Can you work these out from the model? Positions are in its coordinate system, mm. Face numbers are marked on the shaded views. A direction names the side the tool comes from. Round coordinates to 2 decimals unless told otherwise and drop trailing zeros. Loops run counter-clockwise (first coordinate to the right, second up) from the corner with the lowest first, then second, coordinate; pieces in that order, holes last. Notation, with made-up numbers: (-19, -32.5) - (33, -32.5) arc R25 ccw to (33, -9.5) - close; hole circle Ø4 at (-33, 12). An arc over 180 degrees is marked (long way). Answer as CSV lines item,"result".
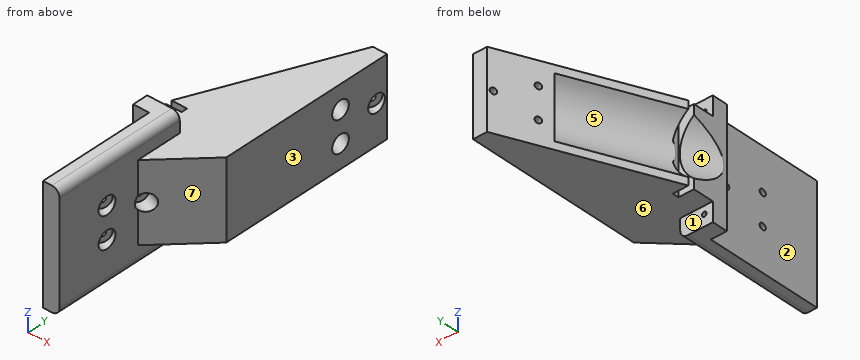
Autodesk Inventor part; units mm, degrees
ref_plane "Work Plane3" through (10.9593, -73.9067, -37.25) normal (-0.9081432, 0.4186597, 0) x (0, 0, 1)
ref_plane "Work Plane4" through (64.6996, 102.2233, -25) normal (-0.9187912, 0.3947439, 0) x (0, 0, 1)
ref_plane "Work Plane5" through (32.5419, 116.0393, -25) normal (-0.9187912, 0.3947439, 0) x (0, 0, 1)
sketch "Sketch1" plane through (0, 0, 0) normal (0, 1, 0) x (-1, 0, 0)
  line L0 (5.5, 37.25) -> (-5.5, 37.25)
  line L1 (-5.5, 37.25) -> (-5.5, -37.25)
  line L2 (-5.5, -37.25) -> (5.5, -37.25)
  line L3 (5.5, -37.25) -> (5.5, 37.25)
  line L4 (5.5, 37.25) -> (-5.5, -37.25) construction
  line L5 (-5.5, 37.25) -> (5.5, -37.25) construction
  circle A0 centre (0, 30) radius 1.5
  line L6 (5.5, 0) -> (-5.5, 0)
  circle A1 centre (0, -30) radius 1.5
  line L7 (-5.5, -25) -> (5.5, -25)
  line L8 (5.5, -25) -> (5.5, 25)
  line L9 (5.5, 25) -> (-5.5, 25)
  line L10 (-5.5, 25) -> (-5.5, -25)
  line L11 (-5.5, -25) -> (5.5, 25) construction
  line L12 (5.5, -25) -> (-5.5, 25) construction
  point P0 (0, 0)
  dimension "d0" = 11
  dimension "d1" = 74.5
  dimension "d2" = 3
  dimension "d3" = 7.25
  dimension "d28" = 50
extrude "Extrusion1" add sketch "Sketch1" along normal blind 10
sketch "Sketch2" plane through (5.5, 0, 37.25) normal (1, 0, 0) x (0, 0, -1)
  line L0 (0, 10) -> (74.5, 10)
  line L1 (0, 0) -> (74.5, 0)
  line L2 (0, 10) -> (74.5, 10)
  line L3 (74.5, 10) -> (74.5, 0)
  line L4 (74.5, 0) -> (0, 0)
  line L5 (0, 0) -> (0, 10)
  point P0 (37.25, 0)
extrude "Extrusion2" add sketch "Sketch2" along normal blind 10
sketch "Sketch3" plane through (0, 0, 0) normal (0, -1, 0) x (1, 0, 0)
  line L0 (-5.5, 37.25) -> (15.5, 37.25)
  line L1 (-5.5, -37.25) -> (15.5, -37.25)
  line L2 (15.5, 37.25) -> (4.8, 37.25)
  line L3 (4.8, 37.25) -> (4.8, -37.25)
  line L4 (4.8, -37.25) -> (15.5, -37.25)
  line L5 (15.5, -37.25) -> (15.5, 37.25)
  point P0 (0, 0)
  dimension "d9" = 10.7
extrude "Extrusion3" add sketch "Sketch3" along normal blind 76
ref_plane "Work Plane1" through (15.5, -76, -37.25) normal (-0.9081432, 0.4186597, 0) x (0, 0, 1)
ref_plane "Work Plane3" through (10.9593, -73.9067, -37.25) normal (-0.9081432, 0.4186597, 0) x (0, 0, 1)
sketch "Sketch4" plane through (10.9593, -73.9067, -37.25) normal (-0.9081432, 0.4186597, 0) x (0, 0, 1)
  circle A0 centre (37.25, 54.5) radius 2
  circle A1 centre (37.25, 54.5) radius 5.5
  circle A2 centre (27.25, 30.8) radius 2
  circle A3 centre (27.25, 30.8) radius 5.5
  line L0 (37.25, 62.5297) -> (37.25, 0)
  line L1 (0, 0) -> (74.5, 0)
  circle A4 centre (47.25, 30.8) radius 5.5
  circle A5 centre (47.25, 30.8) radius 2
  point P0 (37.25, 0)
  dimension "d13" = 4
  dimension "d14" = 11
  dimension "d15" = 4
  dimension "d16" = 11
  dimension "d19" = 10
  dimension "d20" = 23.7
  dimension "d23" = 54.5
extrude "Extrusion4" cut sketch "Sketch4" along normal blind 15 contours A0 L0 | A0 L0 A1 | L0 A0 | A0 L0 A1 | A2 | A3 | A4 | A5
extrude "Extrusion11" cut sketch "Sketch4" along normal blind 25.925 contours A0 L0 | A0 L0 A1 | L0 A0 | A0 L0 A1
extrude "Extrusion6" cut sketch "Sketch4" along normal through all contours A0 L0 | L0 A0 | A2 | A5
extrude "Extrusion7" add sketch "Sketch1" along normal blind 125 contours L3 L6 L1 L9 | L3 L7 L1 L6
sketch "Sketch5" plane through (5.5, 10, -25) normal (1, 0, 0) x (0, 0, -1)
  line L0 (0, 115) -> (-50, 115)
  line L1 (0, 0) -> (0, 115)
  line L2 (-50, 115) -> (0, 115)
  line L3 (0, 115) -> (0, 0)
  line L4 (0, 0) -> (-50, 0)
  line L5 (-50, 0) -> (-50, 115)
  point P0 (-25, -10)
extrude "Extrusion8" add sketch "Sketch5" along normal blind 40
chamfer "Chamfer1" distance 40 angle 23.25 1 edges at (-5.5, 125, 0) measured on face at (-5.5, 48.3333, -8.3333)
sketch "Sketch6" plane through (11.6854, 125, -25) normal (-0.9187912, 0.3947439, 0) x (0, 0, 1)
  circle A0 centre (25, 6.4645) radius 2
  circle A1 centre (25, 6.4645) radius 5.5
  circle A2 centre (15, -17.2355) radius 5.5
  circle A3 centre (15, -17.2355) radius 2
  line L0 (25, 14.6915) -> (25, -47.8381)
  circle A4 centre (35, -17.2355) radius 5.5
  circle A5 centre (35, -17.2355) radius 2
  line L1 (0, -43.5355) -> (50, -43.5355)
  point P0 (25, -119.4616)
  point P1 (25, -43.5355)
  point P2 (25, -43.5355)
  dimension "d36" = 4
  dimension "d37" = 11
  dimension "d38" = 4
  dimension "d39" = 11
  dimension "d40" = 10
  dimension "d41" = 23.7
  dimension "d44" = 50
extrude "Extrusion9" cut sketch "Sketch6" against normal through all contours A0 L0 | L0 A0 | A3 | A5
chamfer "Chamfer2" distance 30 distance2 30 1 edges at (15.5, 10, 0)
sketch "Sketch8" plane through (11.6854, 125, -25) normal (-0.9187912, 0.3947439, 0) x (0, 0, 1)
  line L0 (0, 0) -> (0, 13.3481)
  line L1 (-12.25, -121.6327) -> (62.25, -121.6327)
  line L2 (0, 13.3481) -> (50, 13.3481)
  line L3 (50, 13.3481) -> (50, -121.6327)
  line L4 (50, -121.6327) -> (0, -121.6327)
  line L5 (0, -121.6327) -> (0, 13.3481)
  point P0 (25, -119.4616)
  point P1 (0, 0)
  dimension "d59" = 50
extrude "Extrusion12" cut sketch "Sketch8" against normal blind 22.7
ref_plane "Work Plane4" through (64.6996, 102.2233, -25) normal (-0.9187912, 0.3947439, 0) x (0, 0, 1)
sketch "Sketch9" plane through (64.6996, 102.2233, -25) normal (-0.9187912, 0.3947439, 0) x (0, 0, 1)
  circle A0 centre (35, -17.2355) radius 2
  circle A1 centre (35, -17.2355) radius 5.5
  circle A2 centre (15, -17.2355) radius 2
  circle A3 centre (15, -17.2355) radius 5.5
  circle A4 centre (25, 6.4645) radius 2
  circle A5 centre (25, 6.4645) radius 5.5
  point P0 (25, -119.4616)
  dimension "d63" = 11
  dimension "d64" = 11
  dimension "d65" = 11
extrude "Extrusion13" cut sketch "Sketch9" along normal blind 28.9375 contours A0 | A1 | A2 | A3 | A4 | A5
ref_plane "Work Plane5" through (32.5419, 116.0393, -25) normal (-0.9187912, 0.3947439, 0) x (0, 0, 1)
ref_plane "Work Plane6" through (-5.5, 27.4944, -18.625) normal (0.3947439, 0.9187912, 0) x (0, 0, -1)
sketch "Sketch10" plane through (-5.5, 27.4944, -18.625) normal (0.3947439, 0.9187912, 0) x (0, 0, -1)
  circle A0 centre (-18.625, 15) radius 25
  line L0 (-43.625, 0) -> (6.375, 0)
  point P0 (-18.625, -15.9066)
  point P1 (-38.625, 0)
  point P2 (1.375, 0)
  dimension "d70" = 50
  dimension "d71" = 15
extrude "Extrusion14" cut sketch "Sketch10" along normal blind 70.5 and the other way blind 54.3375
sketch "Sketch11" plane through (15.5, 10, -25) normal (0, 0, -1) x (-1, 0, 0)
  line L0 (21, 17.4944) -> (-6.8294, 82.2691)
  line L1 (21, 17.4944) -> (11, 17.4944)
  line L2 (11, 17.4944) -> (11, 13.4944)
  line L3 (11, 13.4944) -> (21, 13.4944)
  line L4 (21, 13.4944) -> (21, 17.4944)
  point P0 (15.5, -10)
  dimension "d76" = 10
  dimension "d77" = 4
extrude "Extrusion15" cut sketch "Sketch11" against normal blind 70.5
fillet "Fillet1" radius 5 2 edges at (15.5, -33, 37.25) (15.5, -33, -37.25)
properties part number "Camera Bracket"
Q1. We'd pull the mould along Y, two halves only. Please class the marked faces 4, 5, 6 and 7: pulls with the +Y half, pulls with the -Y half, needs draft (parallel to the pull), parting line crosses it, or undercut.
Checks:
face 4,"pulls with the +Y half"
face 5,"undercut"
face 6,"needs draft"
face 7,"pulls with the -Y half"
Q2. If I drill on line 1 along Z through (x, y) = (0, 7); line 2 along X through (y, z) = (23, 18.5); line 3 along Z through (x, y) = (1.5, 38.5), over which ranges is the centre line in solid material (lowest first)? Write a range as [from, to].
Checks:
line 1,"[-37.25, -31.5], [-28.5, 28.5], [31.5, 37.25]"
line 2,"[-5.46, 45.5]"
line 3,"[-25, -18.25], [18.25, 25]"
Q3. Imagine slicing it at B-B (z = 10). Count the separate pieces of the cut face and the enclosed holes in it, then the cut area to 3 significant figures.
Checks:
separate pieces,"3"
enclosed holes,"0"
area,"4,370 mm²"
Q4. On a 3-axis mill with a long thin cutter (end or side, diameter ignored), from which of +Z, -Z, +X, -X, +Y, -Y can I reach the whole of each face in a straight line? I mean the marked faces 1, 2 and 3. Say none if no direction works.
Checks:
face 1,"-Z, +X, -X, +Y"
face 2,"+Z, -Z, -X, -Y"
face 3,"+Z, -Z, +X, +Y, -Y"
Q5. Imagine slicing it at A-A (z = 23). Write out the boundary of the cut face in (x, y), then the cut area to 3 significant figures.
Checks:
outline,"(-5.5, 0) - (4.8, 0) - (4.8, -76) - (15.5, -76) - (15.5, -20) - (45.5, 10) - (45.5, 125) - (36.39, 125) - (-5.5, 27.49) - (4.5, 27.49) - (4.5, 23.49) - (-5.5, 23.49) - close"
area,"5,260 mm²"
Q6. I'm going to push flat-ended pins straight in: pin 1 Ø1 at (x, z) = (22, 19) entering from -Y; pin 2 Ø4 at (x, y) = (13, 70.5) entering from +Z; pin 3 Ø8 at (x, z) = (-0.5, 11.5) entering from -Y. Where does each tip first touch, or does it pass through?
Checks:
pin 1,"y = -14"
pin 2,"z = 25"
pin 3,"y = 0"
